Geometry: final body of the model. Coordinates: model frame, mm. Face numbers are marked on the shaded views. A direction names the side the tool comes from. Give positions to 0.01 mm unless a question says otherwise; leave off trailing zeros. Write each loop counter-clockwise with the first axis right and the second up, starting at its lowest first coordinate (ties: lowest second). Pieces come first, ordered by that corner, then holes. Notation, with made-up numbers: (60, 84) -> (72, 84) arc R31 ccw to (72, 121) -> close; hole circle Ø2 at (-40, -19.75). An arc over 180 degrees is marked (long way). Use CSV: the item, a comma, the result in double quotes. Start each with the question number.
1) Section C-C (x = 16). Output: boundary loops of the cut face in (y, z).
2) Draft query along X for the marked faces 1, 2 and 3. Return one class per face: pulls with the +X half, pulls with the -X half, needs draft (parallel to the pull), parting line crosses it, or undercut.
3) Section B-B (z = 19). Output: boundary loops of the cut face in (x, y), plus the area to 3 significant figures.
4) Set-up query: the marked faces 4, 5, 6, 7 and 8. Return all of +Z, -Z, +X, -X, +Y, -Y with unobstructed straight access to the full face (end or side cutting, diameter ignored); none if empty.
5) Material intervals for line 1 (Z direction, x = 32, y = 3); line 2 (X direction, y = 1.5, z = 17); line 3 (Z direction, x = -4, y = 4.25), sorted ascending. Write a range as [from, to].
6) Section A-A (x = 34). Output: boundary loops of the cut face in (y, z), plus the area to 3 significant figures.
7) Section D-D (z = -6.5). Output: boundary loops of the cut face in (x, y), plus the area to 3 significant figures.
8) Contact query for flat-ended pins moving along their axis: P1, Ø2, axis at x = 6, y = 1, coming from the -Z side; P2, Ø1.9, axis at x = 29.5, y = 3, coming from the +Z side; P3, Ø1.9, axis at x = -17, y = 3, coming from the -Z side; P4, Ø1.5, axis at x = 4.5, y = 5.5, coming from the +Z side. Output: stop coordinate, or through.
```python
from build123d import *

# Parameters (mm, degrees)
SKETCH1_R           = 1.70053
SKETCH1_W           = 19.05
SKETCH1_H           = 25.146
SKETCH1_W_2         = 13.302551819
SKETCH1_H_2         = 6.604
BOSS_EXTRUDE1_DEPTH = 6.35
FILLET8_R           = 2.54


with BuildPart() as part:
    # Sketch1 → Boss-Extrude1 (new body)
    with BuildSketch(Plane(origin=(0, 0, 0), x_dir=(1, 0, 0), z_dir=(0, 1, 0))):
        Polygon((-25.233245497, -25.4), (-6.59007041, -25.4), (-6.59007041, -33.89757), (6.712481409, -33.89757), (6.712481409, -25.4), (25.355656497, -25.4), (38.658208316, -25.4), (41.7070455, -25.4), (41.7070455, 25.4), (38.658208316, 25.4), (25.355656497, 25.4), (6.712481409, 25.4), (6.712481409, 33.89757), (-6.59007041, 33.89757), (-6.59007041, 25.4), (-25.233245497, 25.4), (-38.535797316, 25.4), (-41.5846345, 25.4), (-41.5846345, -25.4), (-38.535797316, -25.4), align=None)
        with Locations(Location((-32.0583645, 10.795, 0), (0, 0, 270))):
            Circle(SKETCH1_R, mode=Mode.SUBTRACT)
        with Locations(Location((-32.0583645, -10.795, 0), (0, 0, 270))):
            Circle(SKETCH1_R, mode=Mode.SUBTRACT)
        with Locations(Location((-6.6583645, -10.795, 0), (0, 0, 270))):
            Circle(SKETCH1_R, mode=Mode.SUBTRACT)
        with Locations(Location((-6.6583645, 10.795, 0), (0, 0, 270))):
            Circle(SKETCH1_R, mode=Mode.SUBTRACT)
        with Locations(Location((0.0612055, -29.81452, 0), (0, 0, 270))):
            Circle(SKETCH1_R, mode=Mode.SUBTRACT)
        with Locations(Location((0.0612055, 29.81452, 0), (0, 0, 270))):
            Circle(SKETCH1_R, mode=Mode.SUBTRACT)
        Polygon((38.658208316, 15.748), (38.658208316, 22.225), (38.658208316, 22.352), (25.355656497, 22.352), (25.355656497, 15.748), align=None, mode=Mode.SUBTRACT)
        with Locations((9.5862055, 0)):
            Rectangle(SKETCH1_W, SKETCH1_H, mode=Mode.SUBTRACT)
        with Locations((0.0612055, -19.05)):
            Rectangle(SKETCH1_W_2, SKETCH1_H_2, mode=Mode.SUBTRACT)
        with Locations((0.0612055, 19.05)):
            Rectangle(SKETCH1_W_2, SKETCH1_H_2, mode=Mode.SUBTRACT)
        Polygon((-38.535797316, 22.352), (-25.233245497, 22.352), (-25.233245497, 22.225), (-25.233245497, 15.748), (-38.535797316, 15.748), align=None, mode=Mode.SUBTRACT)
        with Locations((-31.884521406, -19.05)):
            Rectangle(SKETCH1_W_2, SKETCH1_H_2, mode=Mode.SUBTRACT)
        with Locations((32.006932406, -19.05)):
            Rectangle(SKETCH1_W_2, SKETCH1_H_2, mode=Mode.SUBTRACT)
    extrude(amount=BOSS_EXTRUDE1_DEPTH)

    # Fillet8
    fillet8_edges = [part.edges().sort_by_distance(p)[0] for p in [
        (-6.59007041, 3.175, -25.4),
        (-6.59007041, 3.175, -33.89757),
        (6.712481409, 3.175, -33.89757),
        (6.712481409, 3.175, -25.4),
        (41.7070455, 3.175, -25.4),
        (41.7070455, 3.175, 25.4),
        (6.712481409, 3.175, 25.4),
        (6.712481409, 3.175, 33.89757),
        (-6.59007041, 3.175, 33.89757),
        (-6.59007041, 3.175, 25.4),
        (-41.5846345, 3.175, 25.4),
        (-41.5846345, 3.175, -25.4),
    ]]
    fillet(fillet8_edges, radius=FILLET8_R)


solid = part.part
```
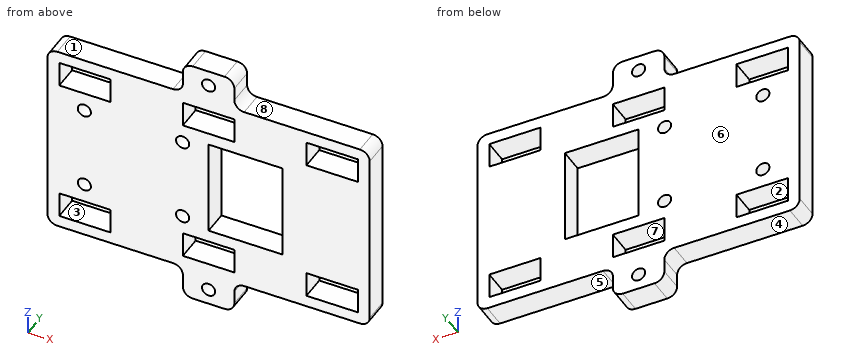
Answers follow:
1,outline,"(0, -25.4) -> (6.35, -25.4) -> (6.35, -12.57) -> (0, -12.57) -> close; (0, 12.57) -> (6.35, 12.57) -> (6.35, 25.4) -> (0, 25.4) -> close"
2,face 1,"needs draft"
2,face 2,"undercut"
2,face 3,"undercut"
3,outline,"(-41.58, 0) -> (-38.54, 0) -> (-38.54, 6.35) -> (-41.58, 6.35) -> close; (-25.23, 0) -> (-6.59, 0) -> (-6.59, 6.35) -> (-25.23, 6.35) -> close; (6.71, 0) -> (25.36, 0) -> (25.36, 6.35) -> (6.71, 6.35) -> close; (38.66, 0) -> (41.71, 0) -> (41.71, 6.35) -> (38.66, 6.35) -> close"
3,area,"275 mm^2"
4,face 4,"-Z, -X, +Y, -Y"
4,face 5,"-Z, +X, +Y, -Y"
4,face 6,"+Z, -Z, +X, -X, +Y"
4,face 7,"+Y, -Y"
4,face 8,"+Z, +X, +Y, -Y"
5,line 1,"z = [-25.4, -22.35], [-15.75, 15.75], [22.35, 25.4]"
5,line 2,"x = [-41.58, -38.54], [-25.23, -6.59], [6.71, 25.36], [38.66, 41.71]"
5,line 3,"z = [-33.9, -22.35], [-15.75, 15.75], [22.35, 33.9]"
6,outline,"(0, -25.4) -> (6.35, -25.4) -> (6.35, -22.35) -> (0, -22.35) -> close; (0, -15.75) -> (6.35, -15.75) -> (6.35, 15.75) -> (0, 15.75) -> close; (0, 22.35) -> (6.35, 22.35) -> (6.35, 25.4) -> (0, 25.4) -> close"
6,area,"239 mm^2"
7,outline,"(-41.58, 0) -> (0.06, 0) -> (0.06, 6.35) -> (-41.58, 6.35) -> close; (19.11, 0) -> (41.71, 0) -> (41.71, 6.35) -> (19.11, 6.35) -> close"
7,area,"408 mm^2"
8,P1,"stops at z = -33.76"
8,P2,"stops at z = 25.4"
8,P3,"stops at z = -25.4"
8,P4,"stops at z = 33.9"
